For this review, take the finished solid that the model builds, in its own axes (mm). Round coordinates to 2 decimals unless told otherwise and drop trailing zeros. Write each loop counter-clockwise with the first axis right and the second up, starting at its lowest first coordinate (ties: lowest second). Pieces come first, ordered by that corner, then holes. Notation, with made-up numbers: M 3,37.25 L 23,37.25 A23 ccw 23,64.25 Z; hole C -37.75,-16.5 d2. An arc over 180 degrees is marked long. Use one line per item in the form item = value. Start each with the question number.
Item 1: Draft analysis for pull direction Y (two halves, no side actions). For faces 1 (the cylindrical face through (26.433, 20.157, 1.014)), 2 (the cylindrical face through (137.167, 17.828, 1.014)), 3 (the flat face through (84, 25, 2)), state which applies: released by +Y, released by -Y, zero draft, split by the parting line, or undercut.
Item 2: Add section B-B (x = 140). State the section outline as (y, z) points, and give its area (3 significant figures).
Item 3: For line 1 (Y direction, x = 140, z = 1.25), list the stretches that pass through material, from the lowest coordinate up. Write a range as [from, to].
Item 4: Add section A-A (y = 20). State the section outline as (x, z) points.
Autodesk Inventor part; units mm, degrees
ref_plane "YZ Plane" through (0, 0, 0) normal (1, 0, 0) x (0, 1, 0)
ref_plane "XZ Plane" through (0, 0, 0) normal (0, 1, 0) x (-1, 0, 0)
ref_plane "XY Plane" through (0, 0, 0) normal (0, 0, 1) x (1, 0, 0)
sketch "Sketch1" plane through (0, 0, 0) normal (0, 0, 1) x (1, 0, 0)
  line L0 (0, 0) -> (170, 0)
  line L1 (170, 0) -> (170, 50)
  line L2 (170, 50) -> (0, 50)
  line L3 (0, 50) -> (0, 0)
  dimension "d0" = 170
  dimension "d1" = 50
extrude "Extrusion1" add sketch "Sketch1" along normal blind 2
sketch "Sketch2" plane through (0, 0, 2) normal (0, 0, 1) x (1, 0, 0)
  circle A0 centre (30, 20) radius 3.57
  circle A1 centre (140, 20) radius 3.57
  line L0 (0, 0) -> (170, 0)
  line L1 (0, 50) -> (0, 0)
  line L2 (170, 0) -> (170, 50)
  dimension "d4" = 7.14
  dimension "d5" = 7.14
  dimension "d6" = 20
  dimension "d7" = 30
  dimension "d8" = 30
  dimension "d9" = 20
extrude "Extrusion2" cut sketch "Sketch2" against normal up to next
properties part number "Panel_5x17cm"
Calculated:
q1.face_1 = undercut
q1.face_2 = undercut
q1.face_3 = zero draft
q2.outline = M 0,0 L 16.43,0 L 16.43,2 L 0,2 Z; M 23.57,0 L 50,0 L 50,2 L 23.57,2 Z
q2.area = 85.7 mm^2
q3.line_1 = [0, 16.43], [23.57, 50]
q4.outline = M 0,0 L 26.43,0 L 26.43,2 L 0,2 Z; M 33.57,0 L 136.43,0 L 136.43,2 L 33.57,2 Z; M 143.57,0 L 170,0 L 170,2 L 143.57,2 Z
